Print and shaded views of the part. All mm, measured from the part's lowest x, y and z. A direction names the side the tool comes from. Give positions to 0.01 mm unless a question says otherwise; leave off trailing zeros. Write each loop counter-clockwise with the first axis right and the second up, starting at its lowest first coordinate (ties: lowest second). Pieces come first, ordered by that corner, then holes. Notation, with made-up numbers: (61.5, 34) -> (120.5, 34) arc R4 ccw to (120.5, 40) -> close; hole circle Ø8 at (46.25, 18). An arc over 180 degrees is marked (long way). Put each result on its own line as item: value.
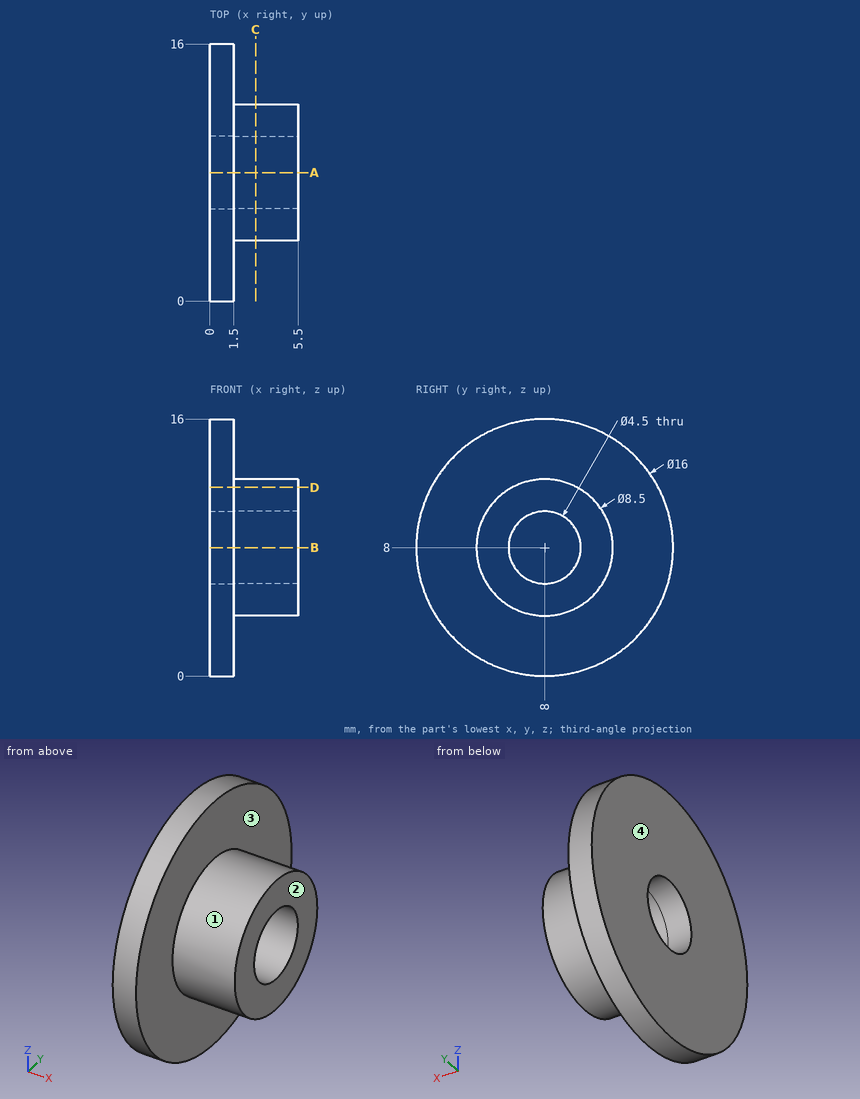
1) Slice it at C-C (x = 2.85). Write the cut outline in (y, z), plus the area to 3 significant figures.
Filled sheet:
outline: circle Ø8.5 at (8, 8); hole circle Ø4.5 at (8, 8)
area: 40.8 mm2
2) Slice it at D-D (z = 11.75). Write the cut outline in (x, y).
Filled sheet:
outline: (0, 0.93) -> (1.5, 0.93) -> (1.5, 6) -> (5.5, 6) -> (5.5, 10) -> (1.5, 10) -> (1.5, 15.07) -> (0, 15.07) -> close
3) Wall check: L1, parallel to Z at x = 3.05, y = 8; L2, parallel to Z at x = 0.95, y = 8; L3, parallel to X at y = 12.5, z = 7.75. Give the ranges that are in metal, low to high.
Filled sheet:
L1: 3.75 to 5.75, 10.25 to 12.25
L2: 0 to 5.75, 10.25 to 16
L3: 0 to 1.5
4) Tool access for the marked faces 3 and 4: list every direction of +Z, -Z, +X, -X, +Y, -Y with a clear straight run to the whole face (end or side of a thin tool).
Filled sheet:
face 3: +X
face 4: +Z, -Z, -X, +Y, -Y
5) Pin check, flat tips, straight feed: pin 1 (1 mm diameter, centred on y = 8, z = 7, fed in from -X); pin 2 (7 mm diameter, centred on y = 8, z = 8, fed in from +X); pin 3 (1 mm diameter, centred on x = 0.5, z = 3, fed in from +Y). Stop position of each tip, or through.
Filled sheet:
pin 1: through
pin 2: x = 5.5
pin 3: y = 14.61
6) Pull direction Z, two halves, no side cores. Call the marked faces 1 and 2: released by +Z, released by -Z, zero draft, split by the parting line, or undercut.
Filled sheet:
face 1: split by the parting line
face 2: zero draft
7) Slice it at A-A (y = 8). Write the cut outline in (x, z).
Filled sheet:
outline: (0, 0) -> (1.5, 0) -> (1.5, 3.75) -> (5.5, 3.75) -> (5.5, 5.75) -> (0, 5.75) -> close; (0, 10.25) -> (5.5, 10.25) -> (5.5, 12.25) -> (1.5, 12.25) -> (1.5, 16) -> (0, 16) -> close
